from build123d import *

# Parameters (mm, degrees)
F0_R     = 9.5
F1_DEPTH = 2
F2_SIZE  = 0.99999
F3_R     = 2.8417127556
F4_DEPTH = 0.6


# Not quite as in the source:
# - a fillet or chamfer is up to 0.001 mm smaller than in the source, because OpenCascade refuses the exact size


with BuildPart() as f1:
    # F0 (on Top) → F1 (new body)
    with BuildSketch(Plane.XY):
        Circle(F0_R)
    extrude(amount=F1_DEPTH)

    # F2 (size 1 in the source; OpenCascade refuses exactly that, so slightly less here)
    f2_edges = [f1.edges().sort_by_distance(p)[0] for p in [
        (-9.5, 0, 2),
        (-9.5, 0, 0),
    ]]
    chamfer(f2_edges, length=F2_SIZE)

    # F3 (on face) → F4 (cut)
    with BuildSketch(Plane.XY.offset(2)):
        with BuildLine():
            ThreePointArc((5.185311865, -1.585620522), (5.4568534532, -0.5346363532), (5.5482306838, 0.5470071919))
            ThreePointArc((5.5482306838, 0.5470071919), (-6.3080923619, 4.0561385788), (1.7284324719, -5.3407049258))
            ThreePointArc((1.7284324719, -5.3407049258), (1.9271777373, -2.0549469321), (5.185311865, -1.585620522))
        make_face()
        with Locations((-0.8992319345, 0.5470071919)):
            Circle(F3_R, mode=Mode.SUBTRACT)
        with BuildLine():
            ThreePointArc((4.9880163164, -2.0816963378), (2.3134948891, -2.4105852235), (2.2065269261, -5.1031287457))
            ThreePointArc((2.2065269261, -5.1031287457), (3.8442696915, -3.8197955903), (4.9880163164, -2.0816963378))
        make_face()
        with BuildLine():
            ThreePointArc((4.9880163164, -2.0816963378), (3.8442696915, -3.8197955903), (2.2065269261, -5.1031287457))
            ThreePointArc((2.2065269261, -5.1031287457), (4.5230773814, -5.7866116654), (5.9249295276, -3.8197955903))
            ThreePointArc((5.9249295276, -3.8197955903), (5.6757845042, -2.8325272153), (4.9880163164, -2.0816963378))
        make_face()
    extrude(amount=-F4_DEPTH, mode=Mode.SUBTRACT)


solid = f1.part
Could you check a few things on this model? Use its own coordinates, in mm. A direction names the side the tool comes from. Round coordinates to 2 decimals unless told otherwise and drop trailing zeros. Write each loop counter-clockwise with the first axis right and the second up, starting at its lowest first coordinate (ties: lowest second). Pieces come first, ordered by that corner, then holes. Notation, with made-up numbers: (48.5, -37) - (68.5, -37) arc R16 ccw to (68.5, -25) - close; hole circle Ø3 at (64.5, 78). An arc over 180 degrees is marked (long way). Use a Markdown table: item, result.
Q1. Please list where these lines run through material, in increasing order: L1, parallel to Y at x = 1.5, z = 1.6; L2, parallel to Y at x = 3.5, z = 1.5; L3, parallel to X at y = -4.5, z = 1.8.
Output values:
| item | result |
|---|---|
| L1 | -8.77 to -5.44, -4.96 to -2.68, -0.98 to 2.07, 6.53 to 8.77 |
| L2 | -8.29 to -5.87, -1.77 to -1.24, 5.26 to 8.29 |
| L3 | -7.45 to -4.91, 1.33 to 1.88, 5.81 to 7.45 |
Q2. For faces 3 (the flat face through (4, -4, 1.4)), 4 (the flat face through (-1, 1, 2)), which set-ups out of +Z, -Z, +X, -X, +Y, -Y let a thin tool reach every point of the face, with its end or its side?
Output values:
| item | result |
|---|---|
| face 3 | +Z |
| face 4 | +Z, +X, -X, +Y, -Y |
Q3. Thinking about a two-plate mould opening in X: for faces 1 (the flat face through (2.5, -1.8, 2)), 2 (the cylindrical face through (1.894, -2.092, 1.704)), which applies, released by +X, released by -X, zero draft, split by the parting line, or undercut?
Output values:
| item | result |
|---|---|
| face 1 | zero draft |
| face 2 | undercut |
Q4. I want a section at B-B (z = 0.7). List the corners of the cut face in (x, y) for me, plus the area to 3 significant figures.
Output values:
| item | result |
|---|---|
| outline | circle Ø18.4 at (0, 0) |
| area | 266 mm2 |
Q5. For pin 1 (1.5 mm diameter, centred on x = -0.5, y = -4, fed in from +Z), with a flat end and sliding along its axis, tell me the tip position at first contact or that it passes through.
Output values:
| item | result |
|---|---|
| pin 1 | z = 1.4 |
